Work out the finished part from the listing and answer in its coordinate system (mm). Face numbers are marked on the shaded views. Round coordinates to 2 decimals unless told otherwise and drop trailing zeros. Order: outer loops, then holes, each group sorted by start corner. A loop starts at its lowest first (then second) coordinate and runs counter-clockwise, first axis right, second up. Notation, with made-up numbers: (-40, 9) - (-22, 9) arc R34 cw to (-22, 46) - close; hole circle Ø1 at (-39, 15). An arc over 180 degrees is marked (long way). Put each result on its own line as item: value.
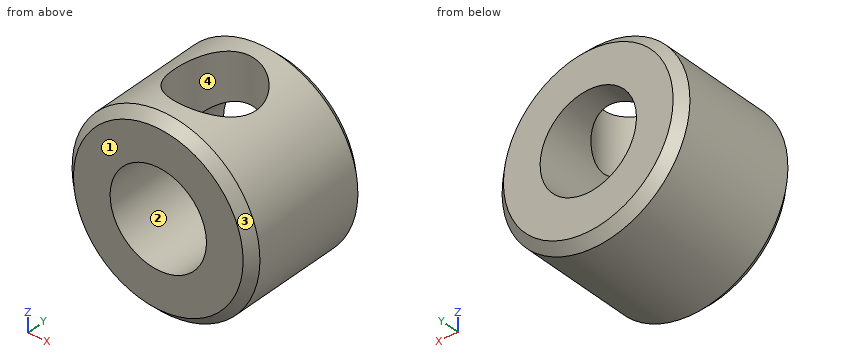
```python
from build123d import *

# Parameters (mm, degrees)
SKETCH1_R                  = 3.937
SKETCH1_R_2                = 2.0193
BOSS_EXTRUDE1_DEPTH        = 5.588
F_8_32_TAPPED_HOLE1_REACH  = 11.236
F_8_32_TAPPED_HOLE1_BORE_R = 1.7272
CHAMFER1_SIZE              = 0.381


with BuildPart() as part:
    # Sketch1 → Boss-Extrude1 (new body)
    with BuildSketch(Plane(origin=(0, 0, 0), x_dir=(1, 0, 0), z_dir=(0, 1, 0))):
        with Locations(Location((0, 0, 0), (0, 0, 270))):
            Circle(SKETCH1_R)
        with Locations(Location((0, 0, 0), (0, 0, 270))):
            Circle(SKETCH1_R_2, mode=Mode.SUBTRACT)
    extrude(amount=BOSS_EXTRUDE1_DEPTH)

    # #8-32 Tapped Hole1 bore (on position points) → #8-32 Tapped Hole1 (cut, up to next)
    with BuildSketch(Plane(origin=(0, 2.794, 3.937), x_dir=(1, 0, 0), z_dir=(0, 0, 1)), mode=Mode.PRIVATE) as f_8_32_tapped_hole1_sk1:
        Circle(F_8_32_TAPPED_HOLE1_BORE_R)
    f_8_32_tapped_hole1_tool1 = extrude(f_8_32_tapped_hole1_sk1.sketch, amount=-F_8_32_TAPPED_HOLE1_REACH, mode=Mode.PRIVATE) & part.part
    add(f_8_32_tapped_hole1_tool1.solids().sort_by_distance((0, 2.794, 3.937))[0], mode=Mode.SUBTRACT)

    # Chamfer1
    chamfer1_edges = [part.edges().sort_by_distance(p)[0] for p in [
        (0, 0, -3.937),
        (0, 5.588, -3.937),
    ]]
    chamfer(chamfer1_edges, length=CHAMFER1_SIZE)


solid = part.part
```
1) A cutting plane is placed at A-A on x = 0. Write down the section's boundary in (y, z).
Findings below:
outline: (0, -3.56) - (0.38, -3.94) - (5.21, -3.94) - (5.59, -3.56) - (5.59, -2.02) - (0, -2.02) - close; (0, 2.02) - (1.07, 2.02) - (1.07, 3.94) - (0.38, 3.94) - (0, 3.56) - close; (4.52, 2.02) - (5.59, 2.02) - (5.59, 3.56) - (5.21, 3.94) - (4.52, 3.94) - close
2) Given pin 1 Ø1.5 at (x, y) = (-2, 2) entering from +Z; pin 2 Ø1.5 at (y, z) = (4.5, -2) entering from +X; pin 3 Ø4 at (x, z) = (0.5, 0.5) entering from -Y; pin 4 Ø3 at (y, z) = (2, 2) entering from -X, each flat-ended and moving along its own axis, determine where each tip first touches the part or whether it passes through.
Findings below:
pin 1: stops at z = 3.71
pin 2: stops at x = 3.73
pin 3: stops at y = 0
pin 4: stops at x = -3.91
3) For a pull along X with two mould halves and no side action, classify the marked faces 1, 2, 3 and 4 as pulls with the +X half, pulls with the -X half, needs draft (parallel to the pull), parting line crosses it, or undercut.
Findings below:
face 1: needs draft
face 2: undercut
face 3: parting line crosses it
face 4: undercut
4) A cutting plane is placed at D-D on y = 2.95. Write down the section's boundary in (x, z).
Findings below:
outline: (-1.72, 1.06) - (-1.72, 3.54) arc R3.94 ccw (long way) to (1.72, 3.54) - (1.72, 1.06) arc R2.02 cw (long way) to start
5) Straight lines are drawn through the part: L1, parallel to X at y = 2.75, z = 0; L2, parallel to Z at x = -0.25, y = 4.65; L3, parallel to X at y = 2, z = 0.75. For each, find the intervals that lie inside material, in ascending order. Write a range as from..to.
Findings below:
L1: x = -3.94..-2.02, 2.02..3.94
L2: z = -3.93..-2, 2..3.93
L3: x = -3.86..-1.87, 1.87..3.86
6) A cutting plane is placed at C-C on y = 1.95. Write down the section's boundary in (x, z).
Findings below:
outline: (-1.51, 1.34) - (-1.51, 3.64) arc R3.94 ccw (long way) to (1.51, 3.64) - (1.51, 1.34) arc R2.02 cw (long way) to start
7) A cutting plane is placed at B-B on z = 0. Write down the section's boundary in (x, y).
Findings below:
outline: (-3.94, 0.38) - (-3.56, 0) - (-2.02, 0) - (-2.02, 5.59) - (-3.56, 5.59) - (-3.94, 5.21) - close; (2.02, 0) - (3.56, 0) - (3.94, 0.38) - (3.94, 5.21) - (3.56, 5.59) - (2.02, 5.59) - close
